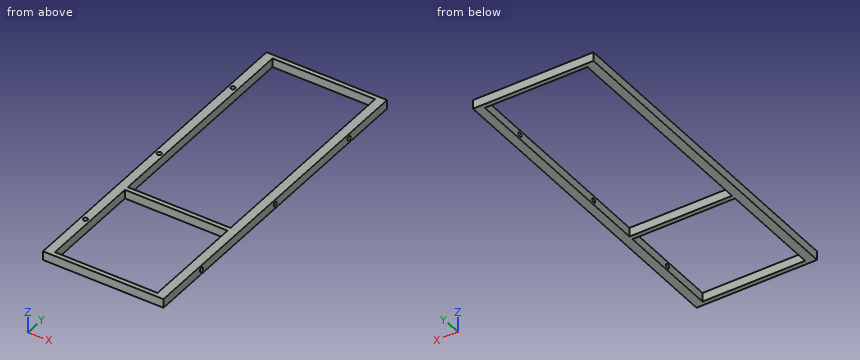
```python
from build123d import *

# Parameters (mm, degrees)
F0_W     = 54
F0_H     = 150
F0_W_2   = 46
F0_H_2   = 47
F0_H_3   = 97
F1_DEPTH = 4
F2_R     = 1
F3_DEPTH = 25
F4_R     = 1
F5_DEPTH = 2


with BuildPart() as f1:
    # F0 (on Top) → F1 (new body)
    with BuildSketch(Plane.XY):
        Rectangle(F0_W, F0_H)
        with Locations((0, -49.5)):
            Rectangle(F0_W_2, F0_H_2, mode=Mode.SUBTRACT)
        with Locations((0, 24.5)):
            Rectangle(F0_W_2, F0_H_3, mode=Mode.SUBTRACT)
    extrude(amount=F1_DEPTH)

    # F2 (on face) → F3 (cut)
    with BuildSketch(Plane.YZ.offset(27)):
        with Locations((-49.5, 2)):
            Circle(F2_R)
        with Locations((0, 2)):
            Circle(F2_R)
        with Locations((49.5, 2)):
            Circle(F2_R)
    extrude(amount=-F3_DEPTH, mode=Mode.SUBTRACT)

    # F4 (on face) → F5 (cut)
    with BuildSketch(Plane.XY.offset(4)):
        with Locations((-25, -49.5)):
            Circle(F4_R)
        with Locations((-25, 0)):
            Circle(F4_R)
        with Locations((-25, 49.5)):
            Circle(F4_R)
    extrude(amount=-F5_DEPTH, mode=Mode.SUBTRACT)


solid = f1.part
```
For this review, take the finished solid that the model builds, in its own axes (mm). Round coordinates to 2 decimals unless told otherwise and drop trailing zeros. Order: outer loops, then holes, each group sorted by start corner. A loop starts at its lowest first (then second) coordinate and runs counter-clockwise, first axis right, second up. Notation, with made-up numbers: (36, -31) -> (71, -31) arc R19 ccw to (71, 3) -> close; hole circle Ø1 at (-17.5, 15). An arc over 180 degrees is marked (long way). Use a Markdown table: item, result.
Item 1: For pin 1 (4 mm diameter, centred on x = 1.5, y = -20.5, fed in from -Z); pin 2 (1.6 mm diameter, centred on y = 49.5, z = 2, fed in from +X), all flat-tipped, find the tip position at first contact; note any pin that passes through.
Resolved:
| item | result |
|---|---|
| pin 1 | passes through |
| pin 2 | stops at x = -23 |
Item 2: For line 1 along Y through (x, z) = (-25, 2.85); line 2 along Y through (x, z) = (15, 0.5); line 3 along X through (y, z) = (-59.5, 1.25), list the stretches that pass through material, from the lowest coordinate up. Write a range as [from, to].
Resolved:
| item | result |
|---|---|
| line 1 | y = [-75, -50.5], [-48.5, -1], [1, 48.5], [50.5, 75] |
| line 2 | y = [-75, -73], [-26, -24], [73, 75] |
| line 3 | x = [-27, -23], [23, 27] |
Item 3: Take a section at A-A (y = 53.5). State the section outline as (x, z) points.
Resolved:
| item | result |
|---|---|
| outline | (-27, 0) -> (-23, 0) -> (-23, 4) -> (-27, 4) -> close; (23, 0) -> (27, 0) -> (27, 4) -> (23, 4) -> close |
